Build history of the part. All positions in model axes, mm. Round coordinates to 2 decimals unless told otherwise and drop trailing zeros. Write each loop counter-clockwise with the first axis right and the second up, starting at its lowest first coordinate (ties: lowest second). Pieces come first, ordered by that corner, then holes.
from build123d import *

# Parameters (mm, degrees)
SKETCH1_R           = 28.65374
SKETCH1_R_2         = 25.2222
BOSS_EXTRUDE1_DEPTH = 69.85
SKETCH1_3_R         = 28.65374
SKETCH1_3_R_2       = 25.2222
BOSS_EXTRUDE2_DEPTH = 11.43
DOME1_FACE_RADIUS   = 28.65374
DOME1_HEIGHT        = 17.78


with BuildPart() as part:
    # Sketch1 → Boss-Extrude1 (new body)
    with BuildSketch(Plane(origin=(0, 0, 0), x_dir=(1, 0, 0), z_dir=(0, 1, 0))):
        with Locations(Location((0, 0, 0), (0, 0, 270))):
            Circle(SKETCH1_R)
        with Locations(Location((0, 0, 0), (0, 0, 270))):
            Circle(SKETCH1_R_2, mode=Mode.SUBTRACT)
    extrude(amount=BOSS_EXTRUDE1_DEPTH)

    # Sketch1<3> → Boss-Extrude2 (add)
    with BuildSketch(Plane(origin=(0, 0, 0), x_dir=(1, 0, 0), z_dir=(0, 1, 0))):
        with Locations(Location((0, 0, 0), (0, 0, 270))):
            Circle(SKETCH1_3_R)
        with Locations(Location((0, 0, 0), (0, 0, 270))):
            Circle(SKETCH1_3_R_2, mode=Mode.SUBTRACT)
        with Locations(Location((0, 0, 0), (0, 0, 270))):
            Circle(SKETCH1_3_R_2)
    extrude(amount=-BOSS_EXTRUDE2_DEPTH)

    # Dome1: a dome of height H over a round flat face of radius A is a cap of a sphere of radius (A * A + H * H) / (2 * H)
    dome1_r = (DOME1_FACE_RADIUS * DOME1_FACE_RADIUS + DOME1_HEIGHT * DOME1_HEIGHT) / (2 * DOME1_HEIGHT)
    dome1_base = Plane((0, -11.43, 0), z_dir=(0, -1, 0))
    with Locations(dome1_base.offset(DOME1_HEIGHT - dome1_r)):
        dome1_ball = Sphere(dome1_r, mode=Mode.PRIVATE)
    add(split(dome1_ball, bisect_by=dome1_base, keep=Keep.TOP, mode=Mode.PRIVATE))


solid = part.part
1) Slice it at B-B (z = 0). Write the cut outline in (x, y), plus the area to 3 significant figures.
Results:
outline: (-28.65, -11.43) arc R31.98 ccw to (28.65, -11.43) - (28.65, 69.85) - (25.22, 69.85) - (25.22, 0) - (-25.22, 0) - (-25.22, 69.85) - (-28.65, 69.85) - close
area: 1,860 mm2
2) Slice it at A-A (x = 0). Write the cut outline in (y, z).
Results:
outline: (-11.43, -28.65) - (69.85, -28.65) - (69.85, -25.22) - (0, -25.22) - (0, 25.22) - (69.85, 25.22) - (69.85, 28.65) - (-11.43, 28.65) arc R31.98 ccw to start
3) Wall check: L1, parallel to Z at x = 0.5, y = 23; L2, parallel to X at y = 46.5, z = 17.5. Give the ranges that are in metal, low to high.
Results:
L1: z = -28.65 to -25.22, 25.22 to 28.65
L2: x = -22.69 to -18.16, 18.16 to 22.69
4) Pin check, flat tips, straight feed: pin 1 Ø25 at (x, z) = (-5, -6) entering from +Y; pin 2 Ø3 at (x, y) = (3.5, -16) entering from +Z; pin 3 Ø6 at (y, z) = (24, -2.5) entering from +X. Stop position of each tip, or through.
Results:
pin 1: stops at y = 0
pin 2: stops at z = 26.7
pin 3: stops at x = 28.65
5) Slice it at C-C (y = 57.5). Write the cut outline in (x, z), plus the area to 3 significant figures.
Results:
outline: circle Ø57.31 at (0, 0); hole circle Ø50.44 at (0, 0)
area: 581 mm2
6) Mould opens along Z. For faces 1 (the cylindrical face through (-17.435, 29.779, -22.739)), 2 (the cylindrical face through (1.1, 34.4, -25.2)), 3 (the flat face through (-25.3, 69.85, 2)) say: released by +Z, released by -Z, zero draft, split by the parting line, or undercut.
Results:
face 1: split by the parting line
face 2: undercut
face 3: zero draft
